Model file for the job. Use its own axes, mm. Coordinates: 2 decimals unless noted, no trailing zeros. Write each loop counter-clockwise with the first axis right and the second up, starting at its lowest first coordinate (ties: lowest second). Pieces come first, ordered by that corner, then holes.
Q1. Band-saw the part on D-D, the plane y = 0.8. State how many separate pieces and enclosed holes the cut face has, plus the area to 3 significant figures.
Q2. Pin check, flat tips, straight feed: P1, Ø4, axis at x = -12.7, z = -30.988, coming from the -Y side; P2, Ø0.7, axis at y = 3.5, z = -24, coming from the -X side; P3, Ø6, axis at x = -50.8, z = -5.588, coming from the -Y side; P4, Ø2, axis at x = -68, y = 1.5, coming from the -Z side. Stop position of each tip, or through.
Q3. Band-saw the part on C-C, the plane x = -63.5. Write the cut outline in (y, z), plus the area to 3 significant figures.
Q4. Band-saw the part on B-B, the plane z = -27.5. Write the cut outline in (x, y), plus the area to 3 significant figures.
Q5. Band-saw the part on A-A, the plane x = -12.7. Write the cut outline in (y, z), plus the area to 3 significant figures.
Q6. Drill centre lines: probe 1 along Z at (x, y) = (-12.7, 1.55); probe 2 along Z at (x, y) = (-63.5, 3.65); probe 3 along Z at (x, y) = (-61.5, 0.6). Where is each one in solid material? Low to high.
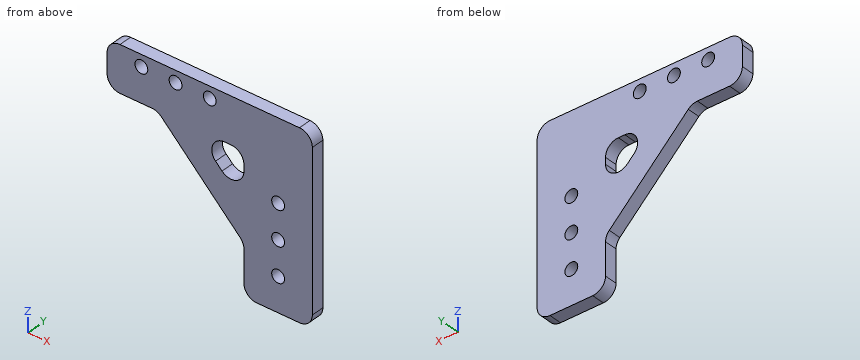
Autodesk Inventor part; units mm, degrees
ref_plane "YZ Plane" through (0, 0, 0) normal (1, 0, 0) x (0, 1, 0)
ref_plane "XZ Plane" through (0, 0, 0) normal (0, 1, 0) x (-1, 0, 0)
ref_plane "XY Plane" through (0, 0, 0) normal (0, 0, 1) x (1, 0, 0)
sketch "Sketch1" plane through (0, 0, 0) normal (0, 1, 0) x (-1, 0, 0)
  line L0 (0, 7.112) -> (15.875, 7.112) construction
  line L1 (20.6375, -69.088) -> (4.7625, -69.088)
  line L2 (0, -64.3255) -> (0, -4.7625)
  line L3 (30.1625, -18.288) -> (76.2, -18.288) construction
  line L4 (76.2, -13.5255) -> (76.2, -4.7625)
  line L5 (71.4375, 0) -> (4.7625, 0)
  line L6 (25.4, -69.088) -> (25.4, -23.0505) construction
  arc A0 (30.1625, -18.288) -> (25.4, -23.0505) centre (30.1625, -23.0505) ccw construction
  arc A1 (0, -64.3255) -> (4.7625, -69.088) centre (4.7625, -64.3255) ccw
  arc A2 (76.2, -4.7625) -> (71.4375, 0) centre (71.4375, -4.7625) ccw
  arc A3 (4.7625, 0) -> (0, -4.7625) centre (4.7625, -4.7625) ccw
  circle A4 centre (12.7, -30.988) radius 2.3876
  circle A5 centre (12.7, -43.688) radius 2.3876
  circle A6 centre (12.7, -56.388) radius 2.3876
  circle A7 centre (63.5, -5.588) radius 2.3876
  circle A8 centre (50.8, -5.588) radius 2.3876
  circle A9 centre (38.1, -5.588) radius 2.3876
  line L7 (76.2, -5.588) -> (0, -5.588) construction
  line L8 (12.7, 0) -> (12.7, -69.088) construction
  line L9 (61.8117, -7.2763) -> (14.3883, -54.6997) construction
  line L10 (56.1403, -19.6829) -> (26.7949, -49.0283)
  line L11 (71.4375, -18.288) -> (59.5079, -18.288)
  line L12 (25.4, -52.3959) -> (25.4, -64.3255)
  arc A10 (71.4375, -18.288) -> (76.2, -13.5255) centre (71.4375, -13.5255) ccw
  arc A11 (20.6375, -69.088) -> (25.4, -64.3255) centre (20.6375, -64.3255) ccw
  arc A12 (59.5079, -18.288) -> (56.1403, -19.6829) centre (59.5079, -23.0505) ccw
  arc A13 (26.7949, -49.0283) -> (25.4, -52.3959) centre (30.1625, -52.3959) ccw
  line L13 (35.9347, -26.4181) -> (33.5301, -28.8227)
  line L14 (25.4, -25.4551) -> (25.4, -23.0505)
  line L15 (32.5671, -18.288) -> (30.1625, -18.288)
  arc A14 (30.1625, -18.288) -> (25.4, -23.0505) centre (30.1625, -23.0505) ccw
  arc A15 (35.9347, -26.4181) -> (32.5671, -18.288) centre (32.5671, -23.0505) ccw
  arc A16 (25.4, -25.4551) -> (33.5301, -28.8227) centre (30.1625, -25.4551) ccw
  point P0 (0, 0)
  point P1 (0, -69.088)
  point P2 (38.1, -5.588)
  point P3 (57.5352, -18.288)
  point P4 (25.4, -50.4232)
  point P5 (44.0648, -18.288)
  point P6 (25.4, -36.9528)
  dimension "d0" = 76.2
  dimension "d1" = 25.4
  dimension "d2" = 4.7625
  dimension "d3" = 4.7752
  dimension "d4" = 12.7
  dimension "d5" = 12.7
  dimension "d6" = 12.7
  dimension "d7" = 12.7
  dimension "d8" = 66.675
  dimension "d9" = 25.4
  dimension "d10" = 38.1
  dimension "d11" = 18.288
  dimension "d12" = 38.1
  dimension "d13" = 12.7
  dimension "d14" = 12.7
  dimension "d15" = 4.7625
  dimension "d16" = 4.7625
  dimension "d17" = 4.7625
  dimension "d18" = 4.7625
extrude "Extrusion1" add sketch "Sketch1" along normal blind 4.7625
thread "Thread1"
thread "Thread2"
thread "Thread3"
thread "Thread4"
thread "Thread5"
thread "Thread6"
sketch "Sketch2" plane through (0, 4.7625, 0) normal (0, 1, 0) x (1, 0, 0)
  line L0 (-71.4375, 0) -> (-4.7625, 0)
  line L1 (-76.2, 1.27) -> (0, 1.27)
  line L2 (-76.2, 13.5255) -> (-76.2, 4.7625)
  line L3 (0, 4.7625) -> (0, 64.3255)
  arc A0 (-4.7625, 0) -> (0, 4.7625) centre (-4.7625, 4.7625) ccw
  line L4 (-4.7625, 0) -> (0, 0)
  line L5 (0, 0) -> (0, 1.27)
  line L6 (-76.2, 1.27) -> (-76.2, 0)
  line L7 (-76.2, 0) -> (-71.4375, 0)
  point P0 (-1.5246, 1.27)
  dimension "d33" = 1.27
extrude "Extrusion2" cut sketch "Sketch2" against normal through all contours L7 L6 L1 A0 L0
fillet "Fillet1" radius 4.7752 2 edges at (-74.6754, 2.3813, -1.27) (-1.5246, 2.3813, -1.27)
properties part number "ELEV_006_SUPBRK1_THRD" material "Aluminum 6061"
Answer sheet:
1. separate pieces: 1
1. enclosed holes: 7
1. area: 2,860 mm2
2. P1: passes through
2. P2: stops at x = -52.17
2. P3: stops at y = 0
2. P4: stops at z = -18.29
3. outline: (0, -18.29) - (4.76, -18.29) - (4.76, -7.98) - (0, -7.98) - close; (0, -3.2) - (4.76, -3.2) - (4.76, -1.27) - (0, -1.27) - close
3. area: 58.3 mm2
4. outline: (-48.32, 0) - (-34.85, 0) - (-34.85, 4.76) - (-48.32, 4.76) - close; (-25.86, 0) - (0, 0) - (0, 4.76) - (-25.86, 4.76) - close
4. area: 187 mm2
5. outline: (0, -69.09) - (4.76, -69.09) - (4.76, -58.78) - (0, -58.78) - close; (0, -54) - (4.76, -54) - (4.76, -46.08) - (0, -46.08) - close; (0, -41.3) - (4.76, -41.3) - (4.76, -33.38) - (0, -33.38) - close; (0, -28.6) - (4.76, -28.6) - (4.76, -1.27) - (0, -1.27) - close
5. area: 255 mm2
6. probe 1: z = -69.09 to -58.78, -54 to -46.08, -41.3 to -33.38, -28.6 to -1.27
6. probe 2: z = -18.29 to -7.98, -3.2 to -1.27
6. probe 3: z = -18.29 to -6.89, -4.28 to -1.27
